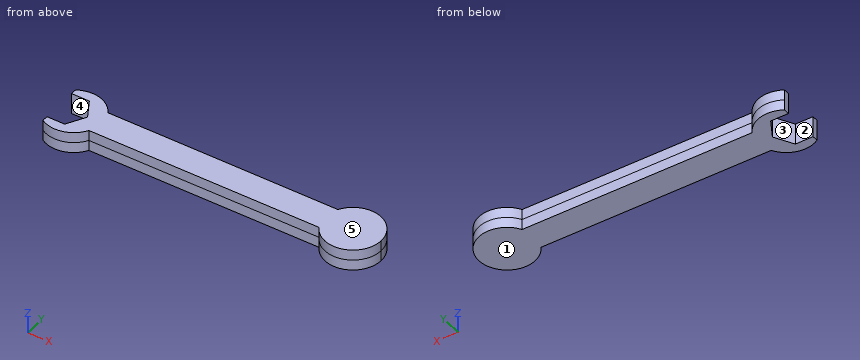
```python
from build123d import *

# Parameters (mm, degrees)
BOSS_EXTRUDE1_DEPTH     = 3.81
CUT_EXTRUDE1_DEPTH      = 111.840048291
CUT_EXTRUDE1_DEPTH_BACK = 111.840048291


with BuildPart() as part:
    # Sketch1 → Boss-Extrude1 (new, symmetric)
    with BuildSketch(Plane.XY):
        with BuildLine():
            ThreePointArc((10.16, 0), (9.813806395, 2.629601498), (8.798818102, 5.08))
            Line((8.798818102, 5.08), (8.798818102, -5.08))
            ThreePointArc((8.798818102, -5.08), (9.813806395, -2.629601498), (10.16, 0))
        make_face()
        with BuildLine():
            Line((8.798818102, -5.08), (8.798818102, 5.08))
            ThreePointArc((8.798818102, 5.08), (-10.16, 0), (8.798818102, -5.08))
        make_face()
        with BuildLine():
            Line((91.348818102, 5.08), (8.798818102, 5.08))
            ThreePointArc((8.798818102, 5.08), (9.813806395, 2.629601498), (10.16, 0))
            ThreePointArc((10.16, 0), (9.813806395, -2.629601498), (8.798818102, -5.08))
            Line((8.798818102, -5.08), (91.348818102, -5.08))
            ThreePointArc((91.348818102, -5.08), (89.987636205, 0), (91.348818102, 5.08))
        make_face()
        with BuildLine():
            ThreePointArc((110.307636205, 0), (102.777237703, 9.813806395), (91.348818102, 5.08))
            Line((91.348818102, 5.08), (91.348818102, -5.08))
            ThreePointArc((91.348818102, -5.08), (102.777237703, -9.813806395), (110.307636205, 0))
        make_face()
        with BuildLine():
            Line((91.348818102, -5.08), (91.348818102, 5.08))
            ThreePointArc((91.348818102, 5.08), (89.987636205, 0), (91.348818102, -5.08))
        make_face()
        with BuildLine():
            ThreePointArc((110.307636205, 0), (102.777237703, 9.813806395), (91.348818102, 5.08))
            Line((91.348818102, 5.08), (91.348818102, -5.08))
            ThreePointArc((91.348818102, -5.08), (102.777237703, -9.813806395), (110.307636205, 0))
        make_face()
        with BuildLine():
            Line((91.348818102, -5.08), (91.348818102, 5.08))
            ThreePointArc((91.348818102, 5.08), (89.987636205, 0), (91.348818102, -5.08))
        make_face()
        with BuildLine():
            ThreePointArc((10.16, 0), (9.813806395, 2.629601498), (8.798818102, 5.08))
            Line((8.798818102, 5.08), (8.798818102, -5.08))
            ThreePointArc((8.798818102, -5.08), (9.813806395, -2.629601498), (10.16, 0))
        make_face()
        with BuildLine():
            Line((8.798818102, -5.08), (8.798818102, 5.08))
            ThreePointArc((8.798818102, 5.08), (-10.16, 0), (8.798818102, -5.08))
        make_face()
    extrude(amount=BOSS_EXTRUDE1_DEPTH, both=True)

    # Sketch2 → Cut-Extrude1 (cut, two sides: drawn at the far end of the back side and taken through both)
    with BuildSketch(Plane.XY.offset(-CUT_EXTRUDE1_DEPTH_BACK)):
        Polygon((1.118947019, 6.599113577), (-5.231052981, 6.599113577), (-5.231052981, -6.599113577), (1.118947019, -6.599113577), (4.928947019, 0), align=None)
        with BuildLine():
            Line((-5.231052981, -6.599113577), (-5.231052981, 6.599113577))
            Line((-5.231052981, 6.599113577), (-6.501052981, 6.599113577))
            Line((-6.501052981, 6.599113577), (-10.156471519, 0.267742946))
            ThreePointArc((-10.156471519, 0.267742946), (-10.16, 0), (-10.156471519, -0.267742946))
            Line((-10.156471519, -0.267742946), (-6.501052981, -6.599113577))
            Line((-6.501052981, -6.599113577), (-5.231052981, -6.599113577))
        make_face()
        with BuildLine():
            Line((-5.231052981, 6.599113577), (-5.231052981, 8.709861349))
            ThreePointArc((-5.231052981, 8.709861349), (-8.775609286, 5.119988443), (-10.156471519, 0.267742946))
            Line((-10.156471519, 0.267742946), (-6.501052981, 6.599113577))
            Line((-6.501052981, 6.599113577), (-5.231052981, 6.599113577))
        make_face()
        with BuildLine():
            Line((-5.231052981, -8.709861349), (-5.231052981, -6.599113577))
            Line((-5.231052981, -6.599113577), (-6.501052981, -6.599113577))
            Line((-6.501052981, -6.599113577), (-10.156471519, -0.267742946))
            ThreePointArc((-10.156471519, -0.267742946), (-8.775609286, -5.119988443), (-5.231052981, -8.709861349))
        make_face()
    extrude(amount=CUT_EXTRUDE1_DEPTH + CUT_EXTRUDE1_DEPTH_BACK, mode=Mode.SUBTRACT)


solid = part.part
```
The listing builds one solid part. Answer for the finished solid, in the listing's coordinates (mm). Face numbers are marked on the shaded views. A direction names the side the tool comes from. Coordinates: 2 decimals unless noted, no trailing zeros. Loops run counter-clockwise (first coordinate to the right, second up) from the corner with the lowest first, then second, coordinate; pieces in that order, holes last. Notation, with made-up numbers: M -25.75,-33.75 L 31.25,-33.75 A10 cw 31.25,-29.75 Z; hole C 23,64 d2. An arc over 180 degrees is marked long. Answer as a JSON object with one key per item and string values. Group by question number.
Item 1: Section C-C (y = -2) is taken. Write down the section's boundary in (x, z).
Item 2: Determine the mould class of the marked faces 1, 2 and 3 for opening direction Y: +Y half, -Y half, draft (parallel to the pull), parting line (faces both ways), or undercut.
Item 3: Consider L1, parallel to Y at x = 64, z = -0.5; L2, parallel to X at y = -5.25, z = 2.25; L3, parallel to X at y = 6.75, z = 2.75. Determine where each line is inside the solid, lowest interval first.
Item 4: Section B-B (x = 47) is taken. Write down the section's boundary in (y, z).
Item 5: Each of these flat-tipped pins is pushed along its axis until it touches: P1, Ø3, axis at x = 66, z = -2.5, coming from the -Y side; P2, Ø4, axis at x = 35.5, z = 2.5, coming from the +Y side; P3, Ø1.5, axis at y = 3, z = -1.5, coming from the -X side. Where does it stop, or does it pass through?
Item 6: Section A-A (z = -1) is taken. Write down the section's boundary in (x, y).
Item 7: Which of the six approach directions +Z, -Z, +X, -X, +Y, -Y give full straight-line access (tool end or side, diameter ignored) to the marked faces 4 and 5?
Solved:
{
 "1": {"outline": "M 3.77,-3.81 L 110.11,-3.81 L 110.11,3.81 L 3.77,3.81 Z"},
 "2": {"face 1": "draft", "face 2": "undercut", "face 3": "undercut"},
 "3": {"L1": "y = -5.08 to 5.08", "L2": "x = 1.9 to 8.7, 91.45 to 108.85", "L3": "x = -5.23 to 7.59, 92.55 to 107.74"},
 "4": {"outline": "M -5.08,-3.81 L 5.08,-3.81 L 5.08,3.81 L -5.08,3.81 Z"},
 "5": {"P1": "stops at y = -5.08", "P2": "stops at y = 5.08", "P3": "stops at x = 2.76"},
 "6": {"outline": "M -5.23,-8.71 A10.16 ccw 8.8,-5.08 L 91.35,-5.08 A10.16 ccw long 91.35,5.08 L 8.8,5.08 A10.16 ccw -5.23,8.71 L -5.23,6.6 L 1.12,6.6 L 4.93,0 L 1.12,-6.6 L -5.23,-6.6 Z"},
 "7": {"face 4": "+Z, -Z, -X", "face 5": "+Z, +X, -X, +Y, -Y"}
}
